```python
from build123d import *

# Parameters (mm, degrees)
SKETCH1_R           = 22
BOSS_EXTRUDE1_DEPTH = 20


with BuildPart() as part:
    # Sketch1 → Boss-Extrude1 (new body)
    # profile 1 of 4: a face of its own
    with BuildSketch(Plane(origin=(0, 0, 0), x_dir=(1, 0, 0), z_dir=(0, 1, 0))):
        with BuildLine():
            Line((-96, -62.5), (96, -62.5))
            Line((96, -62.5), (96, -50.5))
            Line((96, -50.5), (57.998267127, -1.86))
            Line((57.998267127, -1.86), (52.740304928, -6.5))
            Line((52.740304928, -6.5), (32.582594335, 19.300692998))
            Line((32.582594335, 19.300692998), (25.496396068, 28.370613174))
            ThreePointArc((25.496396068, 28.370613174), (22, 31.201938883), (17.616288532, 32.21399842))
            Line((17.616288532, 32.21399842), (-17.616288532, 32.21399842))
            ThreePointArc((-17.616288532, 32.21399842), (-22, 31.201938883), (-25.496396068, 28.370613174))
            Line((-25.496396068, 28.370613174), (-32.582594335, 19.300692998))
            Line((-32.582594335, 19.300692998), (-52.740304928, -6.5))
            Line((-52.740304928, -6.5), (-57.998267127, -1.86))
            Line((-57.998267127, -1.86), (-96, -50.5))
            Line((-96, -50.5), (-96, -62.5))
        make_face()
        with Locations(Location((0, 0, 0), (0, 0, 270))):
            Circle(SKETCH1_R, mode=Mode.SUBTRACT)
    # profile 2 of 4: a face of its own
    with BuildSketch(Plane(origin=(0, 0, 0), x_dir=(1, 0, 0), z_dir=(0, 1, 0))):
        with BuildLine():
            Line((-96, -62.5), (96, -62.5))
            Line((96, -62.5), (96, -50.5))
            Line((96, -50.5), (57.998267127, -1.86))
            Line((57.998267127, -1.86), (52.740304928, -6.5))
            Line((52.740304928, -6.5), (32.582594335, 19.300692998))
            Line((32.582594335, 19.300692998), (25.496396068, 28.370613174))
            ThreePointArc((25.496396068, 28.370613174), (22, 31.201938883), (17.616288532, 32.21399842))
            Line((17.616288532, 32.21399842), (-17.616288532, 32.21399842))
            ThreePointArc((-17.616288532, 32.21399842), (-22, 31.201938883), (-25.496396068, 28.370613174))
            Line((-25.496396068, 28.370613174), (-32.582594335, 19.300692998))
            Line((-32.582594335, 19.300692998), (-52.740304928, -6.5))
            Line((-52.740304928, -6.5), (-57.998267127, -1.86))
            Line((-57.998267127, -1.86), (-96, -50.5))
            Line((-96, -50.5), (-96, -62.5))
        make_face()
        with Locations(Location((0, 0, 0), (0, 0, 270))):
            Circle(SKETCH1_R, mode=Mode.SUBTRACT)
    # profile 3 of 4: a face of its own
    with BuildSketch(Plane(origin=(0, 0, 0), x_dir=(1, 0, 0), z_dir=(0, 1, 0))):
        with BuildLine():
            Line((-96, -62.5), (96, -62.5))
            Line((96, -62.5), (96, -50.5))
            Line((96, -50.5), (57.998267127, -1.86))
            Line((57.998267127, -1.86), (52.740304928, -6.5))
            Line((52.740304928, -6.5), (32.582594335, 19.300692998))
            Line((32.582594335, 19.300692998), (25.496396068, 28.370613174))
            ThreePointArc((25.496396068, 28.370613174), (22, 31.201938883), (17.616288532, 32.21399842))
            Line((17.616288532, 32.21399842), (-17.616288532, 32.21399842))
            ThreePointArc((-17.616288532, 32.21399842), (-22, 31.201938883), (-25.496396068, 28.370613174))
            Line((-25.496396068, 28.370613174), (-32.582594335, 19.300692998))
            Line((-32.582594335, 19.300692998), (-52.740304928, -6.5))
            Line((-52.740304928, -6.5), (-57.998267127, -1.86))
            Line((-57.998267127, -1.86), (-96, -50.5))
            Line((-96, -50.5), (-96, -62.5))
        make_face()
        with Locations(Location((0, 0, 0), (0, 0, 270))):
            Circle(SKETCH1_R, mode=Mode.SUBTRACT)
    # profile 4 of 4: a face of its own
    with BuildSketch(Plane(origin=(0, 0, 0), x_dir=(1, 0, 0), z_dir=(0, 1, 0))):
        with BuildLine():
            Line((-96, -62.5), (96, -62.5))
            Line((96, -62.5), (96, -50.5))
            Line((96, -50.5), (57.998267127, -1.86))
            Line((57.998267127, -1.86), (52.740304928, -6.5))
            Line((52.740304928, -6.5), (32.582594335, 19.300692998))
            Line((32.582594335, 19.300692998), (25.496396068, 28.370613174))
            ThreePointArc((25.496396068, 28.370613174), (22, 31.201938883), (17.616288532, 32.21399842))
            Line((17.616288532, 32.21399842), (-17.616288532, 32.21399842))
            ThreePointArc((-17.616288532, 32.21399842), (-22, 31.201938883), (-25.496396068, 28.370613174))
            Line((-25.496396068, 28.370613174), (-32.582594335, 19.300692998))
            Line((-32.582594335, 19.300692998), (-52.740304928, -6.5))
            Line((-52.740304928, -6.5), (-57.998267127, -1.86))
            Line((-57.998267127, -1.86), (-96, -50.5))
            Line((-96, -50.5), (-96, -62.5))
        make_face()
        with Locations(Location((0, 0, 0), (0, 0, 270))):
            Circle(SKETCH1_R, mode=Mode.SUBTRACT)
    extrude(amount=BOSS_EXTRUDE1_DEPTH)


solid = part.part
```
Can you work these out from the model? Positions are in its coordinate system, mm. A direction names the side the tool comes from. Give positions to 0.01 mm unless a question says otherwise; leave off trailing zeros. Order: outer loops, then holes, each group sorted by start corner. A loop starts at its lowest first (then second) coordinate and runs counter-clockwise, first axis right, second up. Notation, with made-up numbers: M 63.25,23.5 L 74.25,23.5 A36 ccw 74.25,57.5 Z; hole C 7,-4 d6. An arc over 180 degrees is marked long. Write item = value, one per line. Start each with the question number.
Q1. Suppose I cut it at C-C (z = -17.5). Write out the boundary of the cut face in (x, y), plus the area to 3 significant figures.
Q2. I need wall thicknesses on probe 1 along X at (y, z) = (13.25, 10); probe 2 along X at (y, z) = (15, 0); probe 3 along Z at (x, y) = (5.5, 16.5). Which ranges of each line are inside material? Lowest first, please. Write a range as [from, to].
Q3. Suppose I cut it at B-B (y = 15). Write out the boundary of the cut face in (x, z).
Q4. Suppose I cut it at D-D (z = 37). Write out the boundary of the cut face in (x, y).
Q5. Will these pins go through, and if not, where does the flat tip stop? pin 1 Ø1.5 at (y, z) = (8.5, 1) entering from -X; pin 2 Ø1 at (y, z) = (17.5, -7) entering from +X; pin 3 Ø3 at (y, z) = (17.5, 46) entering from -X.
Q6. For faces 1 (the flat face through (55.406, 9.86, 4.148)), 2 (the cylindrical face through (-21.94, 9.86, -31.23)), which set-ups out of +Z, -Z, +X, -X, +Y, -Y let a thin tool reach every point of the face, with its end or its side?
Q7. Suppose I cut it at A-A (x = 0). Write out the boundary of the cut face in (y, z), plus the area to 3 significant figures.
Q8. We'd pull the mould along X, two halves only. Please class faces 3 (the flat face through (-55.332, 9.86, 4.212)), 4 (the flat face through (-96, 10, 56)), 5 (the flat face through (-1, 20, 25)), 6 (the flat face through (96, 10, 57)): pulls with the +X half, pulls with the -X half, needs draft (parallel to the pull), parting line crosses it, or undercut.
Check result:
q1.outline = M -33.99,0 L -13.33,0 L -13.33,20 L -33.99,20 Z; M 13.33,0 L 33.99,0 L 33.99,20 L 13.33,20 Z
q1.area = 826 mm2
q2.probe_1 = [-64.36, -19.6], [19.6, 64.36]
q2.probe_2 = [-47.66, -22], [22, 47.66]
q2.probe_3 = [-32.21, -21.3], [21.3, 62.5]
q3.outline = M -96,50.5 L -58,1.86 L -52.74,6.5 L -25.5,-28.37 A10 ccw -17.62,-32.21 L 17.62,-32.21 A10 ccw 25.5,-28.37 L 52.74,6.5 L 58,1.86 L 96,50.5 L 96,62.5 L -96,62.5 Z; hole C 0,0 d44
q4.outline = M -85.45,0 L 85.45,0 L 85.45,20 L -85.45,20 Z
q5.pin_1 = -49.03
q5.pin_2 = 42.58
q5.pin_3 = -93.66
q6.face_1 = -Z, +Y, -Y
q6.face_2 = -Z, -X, +Y, -Y
q7.outline = M 0,-32.21 L 20,-32.21 L 20,-22 L 0,-22 Z; M 0,22 L 20,22 L 20,62.5 L 0,62.5 Z
q7.area = 1,010 mm2
q8.face_3 = undercut
q8.face_4 = pulls with the -X half
q8.face_5 = needs draft
q8.face_6 = pulls with the +X half
